Part model, mm, in its own coordinate system. Face numbers are marked on the shaded views. A direction names the side the tool comes from. Round coordinates to 2 decimals unless told otherwise and drop trailing zeros. Order: outer loops, then holes, each group sorted by start corner. A loop starts at its lowest first (then second) coordinate and runs counter-clockwise, first axis right, second up. Notation, with made-up numbers: M 2.5,35 L 19.5,35 A17 ccw 19.5,46 Z; hole C 52,-37 d8. An arc over 180 degrees is marked long. One line per question, with ' | ' between items.
from build123d import *

# Parameters (mm, degrees)
SKETCH1_W           = 56.2
SKETCH1_H           = 26.75
SKETCH1_R           = 2.5
SKETCH1_W_2         = 40.2
SKETCH1_H_2         = 20.4
BOSS_EXTRUDE1_DEPTH = 3.175
SKETCH3_W           = 8
SKETCH3_H           = 26.75
BOSS_EXTRUDE2_DEPTH = 20
FILLET1_R           = 4
SKETCH4_R           = 5
BOSS_EXTRUDE3_DEPTH = 40


with BuildPart() as part:
    # Sketch1 → Boss-Extrude1 (new body)
    with BuildSketch(Plane(origin=(0, 0, 0), x_dir=(1, 0, 0), z_dir=(0, 1, 0))):
        Rectangle(SKETCH1_W, SKETCH1_H)
        with Locations(Location((24.8, 5, 0), (0, 0, 270))):
            Circle(SKETCH1_R, mode=Mode.SUBTRACT)
        with Locations(Location((24.8, -5, 0), (0, 0, 270))):
            Circle(SKETCH1_R, mode=Mode.SUBTRACT)
        with Locations(Location((-24.8, -5, 0), (0, 0, 90))):
            Circle(SKETCH1_R, mode=Mode.SUBTRACT)
        with Locations(Location((-24.8, 5, 0), (0, 0, 90))):
            Circle(SKETCH1_R, mode=Mode.SUBTRACT)
        Rectangle(SKETCH1_W_2, SKETCH1_H_2, mode=Mode.SUBTRACT)
    extrude(amount=BOSS_EXTRUDE1_DEPTH)

    # Sketch3 → Boss-Extrude2 (add)
    with BuildSketch(Plane.XZ):
        with Locations((24.1, 0)):
            Rectangle(SKETCH3_W, SKETCH3_H)
    extrude(amount=BOSS_EXTRUDE2_DEPTH)

    # Fillet1
    fillet1_edges = [part.edges().sort_by_distance(p)[0] for p in [
        (28.1, -8.4125, 13.375),
        (-28.1, 1.5875, 13.375),
        (-28.1, 1.5875, -13.375),
        (28.1, -8.4125, -13.375),
    ]]
    fillet(fillet1_edges, radius=FILLET1_R)

    # Sketch4 → Boss-Extrude3 (add)
    with BuildSketch(Plane(origin=(28.1, 0, 0), x_dir=(0, 0, -1), z_dir=(1, 0, 0))):
        with Locations(Location((0, -11.825, 0), (0, 0, 180))):
            Circle(SKETCH4_R)
    extrude(amount=BOSS_EXTRUDE3_DEPTH)


solid = part.part
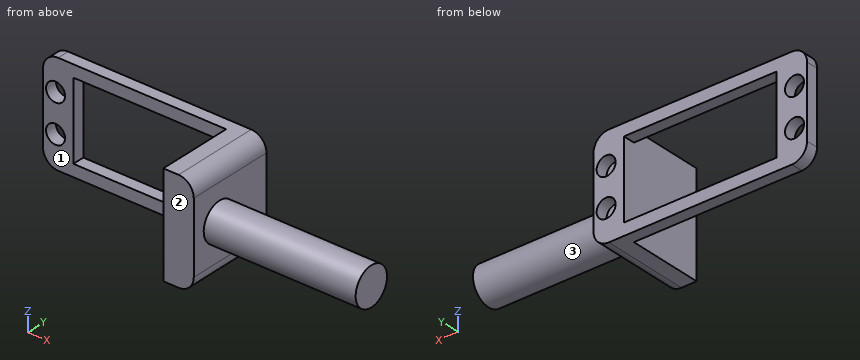
1) Saw through at D-D (z = 4). List the corners of the cut face in (x, y) (3 decimals).
The answers:
outline: M -28.1,0 L -27.091,0 L -27.091,3.175 L -28.1,3.175 Z; M -22.509,0 L -20.1,0 L -20.1,3.175 L -22.509,3.175 Z; M 20.1,-20 L 28.1,-20 L 28.1,-14.825 L 68.1,-14.825 L 68.1,-8.825 L 28.1,-8.825 L 28.1,3.175 L 27.091,3.175 L 27.091,0 L 22.509,0 L 22.509,3.175 L 20.1,3.175 Z
2) Saw through at C-C (y = -8.25). List the corners of the cut face in (x, z) (3 decimals).
The answers:
outline: M 20.1,-13.375 L 24.1,-13.375 A4 ccw 28.1,-9.375 L 28.1,-3.496 L 68.1,-3.496 L 68.1,3.496 L 28.1,3.496 L 28.1,9.375 A4 ccw 24.1,13.375 L 20.1,13.375 Z
3) Which spindle directions (+Z, -Z, +X, -X, +Y, -Y) get a long thin tool onto all of the face, cutting with end or side? Do the marked faces 1, 2 and 3. Say none if no direction does.
The answers:
face 1: +Z, -Z, -X, -Y | face 2: +Z, -Z, +X, -X, -Y | face 3: +X
4) Saw through at A-A (z = 0). List the corners of the cut face in (x, y) (3 decimals).
The answers:
outline: M -28.1,0 L -20.1,0 L -20.1,3.175 L -28.1,3.175 Z; M 20.1,-20 L 28.1,-20 L 28.1,-16.825 L 68.1,-16.825 L 68.1,-6.825 L 28.1,-6.825 L 28.1,3.175 L 20.1,3.175 Z
5) Probe line 1 (X direction, y = 0.9, z = -5); line 2 (Z direction, x = -24.8, y = 1.2); line 3 (Z direction, x = 13.5, y = 1.5) (3 decimals). List the from-to ranges inside material, lowest first. Write a range as [from, to].
The answers:
line 1: x = [-28.1, -27.3], [-22.3, -20.1], [20.1, 22.3], [27.3, 28.1] | line 2: z = [-13.31, -7.5], [-2.5, 2.5], [7.5, 13.31] | line 3: z = [-13.375, -10.2], [10.2, 13.375]
6) Saw through at B-B (x = -16.5). List the corners of the cut face in (y, z) (3 decimals).
The answers:
outline: M 0,-13.375 L 3.175,-13.375 L 3.175,-10.2 L 0,-10.2 Z; M 0,10.2 L 3.175,10.2 L 3.175,13.375 L 0,13.375 Z
7) Drop flat-ended pins along their axis: pin 1 (1.6 mm diameter, centred on y = 2, z = -1.5, fed in from +X); pin 2 (4 mm diameter, centred on x = 25, z = -5, fed in from +Y); pin 3 (3 mm diameter, centred on x = -15.5, z = -10, fed in from +Y) (3 decimals); pin 4 (3 mm diameter, centred on y = -14.5, z = -6, fed in from -X). Give the stop position or say it passes through.
The answers:
pin 1: stops at x = 28.1 | pin 2: stops at y = 0 | pin 3: stops at y = 3.175 | pin 4: stops at x = 20.1
